Check sheet for the modelled part. Datum: model origin and axes. Units: mm. A direction names the side the tool comes from. Give positions to 0.01 mm unless a question says otherwise; leave off trailing zeros. Loops run counter-clockwise (first coordinate to the right, second up) from the corner with the lowest first, then second, coordinate; pieces in that order, holes last. Notation, with made-up numbers: M -21,8 L 7,8 A12 cw 7,19 Z; hole C -33,46 d5. An arc over 180 degrees is marked long. Use one line per item in the form item = value.
Autodesk Fusion 360 part; units mm, degrees
sketch "Esquisse1" plane through (0, 0, 0) normal (0, 0, 1) x (1, 0, 0)
  circle A0 centre (0, 0) radius 16.55
  circle A1 centre (0, 0) radius 4.1
  circle A2 centre (-13, 0) radius 2
  circle A3 centre (0, -13) radius 2
  circle A4 centre (13, 0) radius 2
  circle A5 centre (0, 13) radius 2
  dimension "d1" = 33.1
  dimension "d2" = 8.2
  dimension "d3" = 4
  dimension "d4" = 13
  dimension "d6" = 360
extrude "Extrusion1" add sketch "Esquisse1" along normal blind 19
sketch "Esquisse2" plane through (0, 0, 0) normal (0, 0, -1) x (1, 0, 0)
  circle A0 centre (13, 0) radius 2
  circle A1 centre (-13, 0) radius 2
  circle A2 centre (0, 0) radius 4.1
  circle A3 centre (0, 13) radius 2
  circle A4 centre (0, -13) radius 2
  circle A5 centre (0, 0) radius 16.55
hole "Perçage1" at (0, -13, 0) direction (0, 0, 1) diameter 6 depth 4 tip angle 180
hole "Perçage2" at (-13, 0, 0) direction (0, 0, 1) diameter 6 depth 4 tip angle 180
hole "Perçage3" at (13, 0, 0) direction (0, 0, 1) diameter 6 depth 4 tip angle 180
hole "Perçage4" at (0, 13, 0) direction (0, 0, 1) diameter 6 depth 4 tip angle 180
hole "Perçage5" at (0, 0, 19) direction (0, 0, -1) diameter 22.5 depth 2 tip angle 180
sketch "Esquisse3" plane through (0, 0, 19) normal (0, 0, 1) x (-1, 0, 0)
  circle A0 centre (0, 0) radius 16.55
  arc A1 (11.2139, 0.9) -> (0.9, 11.2139) centre (0, 0) ccw
  arc A2 (11.2139, -0.9) -> (11.2139, 0.9) centre (13, 0) ccw
  arc A3 (0.9, -11.2139) -> (11.2139, -0.9) centre (0, 0) ccw
  arc A4 (-0.9, -11.2139) -> (0.9, -11.2139) centre (0, -13) ccw
  arc A5 (-11.2139, -0.9) -> (-0.9, -11.2139) centre (0, 0) ccw
  arc A6 (-11.2139, 0.9) -> (-11.2139, -0.9) centre (-13, 0) ccw
  arc A7 (-0.9, 11.2139) -> (-11.2139, 0.9) centre (0, 0) ccw
  arc A8 (0.9, 11.2139) -> (-0.9, 11.2139) centre (0, 13) ccw
  circle A9 centre (0, 0) radius 20
  dimension "d24" = 40
extrude "Extrusion2" add sketch "Esquisse3" against normal blind 7.1 contours A9
sketch "Esquisse4" plane through (0, 0, 19) normal (0, 0, 1) x (-1, 0, 0)
  circle A0 centre (0, 0) radius 20
  arc A1 (11.2139, 0.9) -> (0.9, 11.2139) centre (0, 0) ccw
  arc A2 (11.2139, -0.9) -> (11.2139, 0.9) centre (13, 0) ccw
  arc A3 (0.9, -11.2139) -> (11.2139, -0.9) centre (0, 0) ccw
  arc A4 (-0.9, -11.2139) -> (0.9, -11.2139) centre (0, -13) ccw
  arc A5 (-11.2139, -0.9) -> (-0.9, -11.2139) centre (0, 0) ccw
  arc A6 (-11.2139, 0.9) -> (-11.2139, -0.9) centre (-13, 0) ccw
  arc A7 (-0.9, 11.2139) -> (-11.2139, 0.9) centre (0, 0) ccw
  arc A8 (0.9, 11.2139) -> (-0.9, 11.2139) centre (0, 13) ccw
  line L0 (0, 0) -> (14.1421, -14.1421) construction
  line L1 (0, 0) -> (20, 0) construction
  line L2 (0, 0) -> (18.7939, -6.8404) construction
  line L3 (0, 0) -> (6.8404, -18.7939) construction
  line L4 (0, 0) -> (20, 0) construction
  line L5 (18.7939, -6.8404) -> (10.5715, -3.8477)
  line L6 (6.8404, -18.7939) -> (3.8477, -10.5715)
  arc A9 (3.8477, -10.5715) -> (10.5715, -3.8477) centre (0, 0) ccw
  arc A10 (6.8404, -18.7939) -> (18.7939, -6.8404) centre (0, 0) ccw
  arc A11 (10.5715, 3.8477) -> (3.8477, 10.5715) centre (0, 0) ccw
  line L7 (6.8404, 18.7939) -> (3.8477, 10.5715)
  arc A12 (18.7939, 6.8404) -> (6.8404, 18.7939) centre (0, 0) ccw
  line L8 (18.7939, 6.8404) -> (10.5715, 3.8477)
  arc A13 (-3.8477, 10.5715) -> (-10.5715, 3.8477) centre (0, 0) ccw
  line L9 (-18.7939, 6.8404) -> (-10.5715, 3.8477)
  arc A14 (-6.8404, 18.7939) -> (-18.7939, 6.8404) centre (0, 0) ccw
  line L10 (-6.8404, 18.7939) -> (-3.8477, 10.5715)
  arc A15 (-10.5715, -3.8477) -> (-3.8477, -10.5715) centre (0, 0) ccw
  line L11 (-6.8404, -18.7939) -> (-3.8477, -10.5715)
  arc A16 (-18.7939, -6.8404) -> (-6.8404, -18.7939) centre (0, 0) ccw
  line L12 (-18.7939, -6.8404) -> (-10.5715, -3.8477)
  dimension "d27" = 45
  dimension "d28" = 25
  dimension "d29" = 70
  dimension "d31" = 360
extrude "Extrusion3" add sketch "Esquisse4" along normal blind 5 contours A0 A1 A11 L7 A12 L8 | A0 A3 L5 L6 A9 A10 | A0 A7 A13 L9 A14 L10 | A0 A5 A15 L11 A16 L12
1) Section check D-D (z = 22.25). Record the cut outline in (x, y).
Evaluation:
outline = M -18.79,-6.84 A20 ccw -6.84,-18.79 L -3.85,-10.57 A11.25 cw -10.57,-3.85 Z; M -18.79,6.84 L -10.57,3.85 A11.25 cw -3.85,10.57 L -6.84,18.79 A20 ccw Z; M 3.85,-10.57 L 6.84,-18.79 A20 ccw 18.79,-6.84 L 10.57,-3.85 A11.25 cw Z; M 3.85,10.57 A11.25 cw 10.57,3.85 L 18.79,6.84 A20 ccw 6.84,18.79 Z
2) Depth check by flat-ended pin: pin 1 Ø2 at (x, z) = (8.5, 18) entering from -Y; pin 2 Ø11 at (x, y) = (-4.5, -0.5) entering from +Z; pin 3 Ø3 at (y, z) = (-13.5, 13.5) entering from +X. Enter the tip coordinate at first touch or a pass-through.
Evaluation:
pin_1 = -18.54
pin_2 = 17
pin_3 = 16
3) Section check A-A (y = 0). Record the cut outline in (x, z), then the cut area to 3 significant figures.
Evaluation:
outline = M -20,11.9 L -16.55,11.9 L -16.55,0 L -16,0 L -16,4 L -15,4 L -15,19 L -20,19 Z; M -11,4 L -10,4 L -10,0 L -4.1,0 L -4.1,17 L -11,17 Z; M 4.1,0 L 10,0 L 10,4 L 11,4 L 11,17 L 4.1,17 Z; M 15,4 L 16,4 L 16,0 L 16.55,0 L 16.55,11.9 L 20,11.9 L 20,19 L 15,19 Z
area = 326 mm^2
4) Scan lines: line 1 (Y direction, x = 0, z = 14); line 2 (Y direction, x = 0, z = 11). Record each from-to range of solid material in increasing order.
Evaluation:
line_1 = -20 to -15, -11 to -4.1, 4.1 to 11, 15 to 20
line_2 = -16.55 to -15, -11 to -4.1, 4.1 to 11, 15 to 16.55
5) Section check C-C (z = 8.25). Record the cut outline in (x, y), then the cut area to 3 significant figures.
Evaluation:
outline = C 0,0 d33.1; hole C -13,0 d4; hole C 0,0 d8.2; hole C 0,-13 d4; hole C 0,13 d4; hole C 13,0 d4
area = 757 mm^2
6) Release check for a two-part mould opening along X. For faces 4 (the face through (-9.229, 17.743, 16.69)), 5 (the face through (15.93, -0.65, 2.03)), 6 (the face through (3.4, -3.4, 0)) record: pulls with the +X half, pulls with the -X half, needs draft (parallel to the pull), parting line crosses it, or undercut.
Evaluation:
face_4 = parting line crosses it
face_5 = undercut
face_6 = needs draft
7) Set-up check for faces 1 (the face through (-16, 0, 19)), 2 (the face through (15, 1, 4)), 3 (the face through (16, 0, 19)): record each of +Z, -Z, +X, -X, +Y, -Y from which the full face is reachable in a straight line by a thin tool's end or side.
Evaluation:
face_1 = +Z, -X
face_2 = -Z
face_3 = +Z, +X
